Geometry: final body of the model. Coordinates: model frame, mm. Coordinates: 2 decimals unless noted, no trailing zeros. Write each loop counter-clockwise with the first axis right and the second up, starting at its lowest first coordinate (ties: lowest second). Pieces come first, ordered by that corner, then holes.
Solid Edge part; units mm, degrees
sketch "Sketch1" plane through (0, 0, 0) normal (0, 0, 1) x (1, 0, 0)
  line L0 (45, -45) -> (-45, -45)
  line L1 (-45, -45) -> (-45, 45)
  line L2 (-45, 45) -> (45, 45)
  line L3 (45, 45) -> (45, -45)
  dimension "D1" = 45
  dimension "D2" = 45
extrude "Protrusion1" add sketch "Sketch1" along normal blind 3
hole "Hole_3" at (-40, 40, 3) direction (0, 0, -1) diameter 3.2 end through all
hole "Hole1" at (-40, -40, 3) direction (0, 0, -1) diameter 3.2 end through all
hole "Hole2" at (40, -40, 3) direction (0, 0, -1) diameter 3.2 end through all
hole "Hole3" at (40, 40, 3) direction (0, 0, -1) diameter 3.2 end through all
hole "Hole4" at (-31.82, 0, 3) direction (0, 0, -1) diameter 4.2 end through all
hole "Hole5" at (0, 31.8196, 3) direction (0, 0, -1) diameter 4.2 end through all
hole "Hole6" at (31.82, 0, 3) direction (0, 0, -1) diameter 4.2 end through all
hole "Hole7" at (0, -31.8196, 3) direction (0, 0, -1) diameter 4.2 end through all
hole "Hole_11" at (0, 0, 3) direction (0, 0, -1) diameter 4.134 end up to next thread major 5 thread length 2
hole "Hole_16" at (-15, -35, 3) direction (0, 0, -1) diameter 4 end up to next
hole "Hole8" at (15, -35, 3) direction (0, 0, -1) diameter 4 end up to next
pattern_circular "Pattern2" count 4 over 360 about axis through (0, 0, 3) along (0, 0, -1) of "Hole_16", "Hole8"
properties material "アルミニウム, 5050"
Item 1: Section C-C, the plane x = 0. Output: boundary loops of the cut face in (y, z).
Derived:
outline: (-45, 0) - (-33.92, 0) - (-33.92, 3) - (-45, 3) - close; (-29.72, 0) - (-2.07, 0) - (-2.07, 3) - (-29.72, 3) - close; (2.07, 0) - (29.72, 0) - (29.72, 3) - (2.07, 3) - close; (33.92, 0) - (45, 0) - (45, 3) - (33.92, 3) - close
Item 2: Pin query (flat end, axial travel): pin 1 (5 mm diameter, centred on x = 15, y = -35, fed in from +Z); pin 2 (3.5 mm diameter, centred on x = 0, y = 0, fed in from +Z). Return the tip coordinate at first contact, or that it passes through.
Derived:
pin 1: stops at z = 3
pin 2: passes through
Item 3: Section A-A, the plane x = 35. Output: boundary loops of the cut face in (y, z).
Derived:
outline: (-45, 0) - (-17, 0) - (-17, 3) - (-45, 3) - close; (-13, 0) - (13, 0) - (13, 3) - (-13, 3) - close; (17, 0) - (45, 0) - (45, 3) - (17, 3) - close
Item 4: Pull-direction query (Y, two-part tool) for faces 1 (the cylindrical face through (36.908, 15.601, 1.521)), 2 (the cylindrical face through (-1.26, 1.64, 1.52)), 3 (the flat face through (-1, 45, 1)), 4 (the flat face through (45, 1, 1)); classes: released by +Y, released by -Y, zero draft, split by the parting line, or undercut.
Derived:
face 1: undercut
face 2: undercut
face 3: released by +Y
face 4: zero draft
Item 5: Material intervals for probe 1 along Y at (x, z) = (-35, 1.7); probe 2 along Y at (x, z) = (0, 2.25), sorted ascending.
Derived:
probe 1: y = -45 to -17, -13 to 13, 17 to 45
probe 2: y = -45 to -33.92, -29.72 to -2.07, 2.07 to 29.72, 33.92 to 45
Item 6: Section D-D, the plane z = 0.8. State how many separate pieces and enclosed holes the cut face has, plus the area to 3 significant figures.
Derived:
separate pieces: 1
enclosed holes: 17
area: 7,900 mm2
